```python
from build123d import *

# Parameters (mm, degrees)
BOSS_EXTRUDE1_DEPTH     = 5
CUT_EXTRUDE1_DEPTH      = 151.083310198
CUT_EXTRUDE1_DEPTH_BACK = 151.083310198
SKETCH2_R               = 4
SKETCH2_R_2             = 2.665209895


with BuildPart() as part:
    # Sketch1 → Boss-Extrude1 (new body)
    with BuildSketch(Plane(origin=(0, 0, 0), x_dir=(1, 0, 0), z_dir=(0, 1, 0))):
        Polygon((0, 129.903810568), (75, 0), (-75, 0), align=None)
    extrude(amount=BOSS_EXTRUDE1_DEPTH)

    # Sketch2 → Cut-Extrude1 (cut, two sides: drawn at the far end of the back side and taken through both)
    with BuildSketch(Plane(origin=(0, 5, 0), x_dir=(1, 0, 0), z_dir=(0, 1, 0)).offset(-CUT_EXTRUDE1_DEPTH_BACK)):
        with Locations(Location((-61.143593539, 8, 0), (0, 0, 270))):
            Circle(SKETCH2_R)
        with Locations(Location((61.143593539, 8, 0), (0, 0, 270))):
            Circle(SKETCH2_R)
        with Locations(Location((0, 113.903810568, 0), (0, 0, 270))):
            Circle(SKETCH2_R)
        with Locations(Location((0, 43.301270189, 0), (0, 0, 270))):
            Circle(SKETCH2_R_2)
    extrude(amount=CUT_EXTRUDE1_DEPTH + CUT_EXTRUDE1_DEPTH_BACK, mode=Mode.SUBTRACT)


solid = part.part
```
Geometry check sheet. Reference: the model listing, model coordinates, mm. Give positions to 0.01 mm unless a question says otherwise; leave off trailing zeros. Write each loop counter-clockwise with the first axis right and the second up, starting at its lowest first coordinate (ties: lowest second). Pieces come first, ordered by that corner, then holes.
1) Section check B-B, the plane y = 2.5. Record the boundary of the cut face in (x, z), and give its area (3 significant figures).
2) Section check D-D, the plane x = -55.5. Record the boundary of the cut face in (y, z) (3 decimals).
3) Material ranges on L1, parallel to Z at x = 0, y = 3.5; L2, parallel to X at y = 2.75, z = -8; L3, parallel to X at y = 3.6, z = -44, recorded low to high.
4) Gauge pin test, flat ends, axial feed: pin 1 (1.5 mm diameter, centred on y = 2, z = -44.5, fed in from +X); pin 2 (7 mm diameter, centred on x = 0, z = -113.9, fed in from -Y); pin 3 (2 mm diameter, centred on y = 4.5, z = -93.5, fed in from -X). Record the tip position at first contact, or that the pin passes through.
5) Section check A-A, the plane z = -7.5. Record the boundary of the cut face in (x, y).
6) Release check for a two-part mould opening along X. For faces 1 (the cylindrical face through (-65.048, 2.465, -8.867)), 2 (the flat face through (1, 2, 0)), 3 (the cylindrical face through (1.801, 2.465, -45.266)), 4 (the flat face through (36.975, 2.465, -65.861)) record: pulls with the +X half, pulls with the -X half, needs draft (parallel to the pull), parting line crosses it, or undercut.
7) Section check C-C, the plane z = -112. Record the boundary of the cut face in (x, y).
Computed:
1. outline: (-75, 0) - (0, -129.9) - (75, 0) - close; hole circle Ø8 at (-61.14, -8); hole circle Ø8 at (0, -113.9); hole circle Ø5.33 at (0, -43.3); hole circle Ø8 at (61.14, -8)
1. area: 9,570 mm2
2. outline: (0, -33.775) - (5, -33.775) - (5, 0) - (0, 0) - close
3. L1: z = -129.9 to -117.9, -109.9 to -45.97, -40.64 to 0
3. L2: x = -70.38 to -65.14, -57.14 to 57.14, 65.14 to 70.38
3. L3: x = -49.6 to -2.57, 2.57 to 49.6
4. pin 1: stops at x = 49.74
4. pin 2: passes through
4. pin 3: stops at x = -21.6
5. outline: (-70.67, 0) - (-65.11, 0) - (-65.11, 5) - (-70.67, 5) - close; (-57.17, 0) - (57.17, 0) - (57.17, 5) - (-57.17, 5) - close; (65.11, 0) - (70.67, 0) - (70.67, 5) - (65.11, 5) - close
6. face 1: undercut
6. face 2: needs draft
6. face 3: undercut
6. face 4: pulls with the +X half
7. outline: (-10.34, 0) - (-3.52, 0) - (-3.52, 5) - (-10.34, 5) - close; (3.52, 0) - (10.34, 0) - (10.34, 5) - (3.52, 5) - close
